```python
from build123d import *

# Parameters (mm, degrees)
F0_R     = 5.5
F0_R_2   = 3.25
F1_DEPTH = 30
F2_R     = 2.75
F2_R_2   = 1.75
F2_R_3   = 3.5
F2_R_4   = 8.25
F2_R_5   = 12.5
F3_DEPTH = 5
F5_DEPTH = 28
F7_DEPTH = 25
F8_SIZE  = 2


with BuildPart() as f1:
    # F0 (on Front) → F1 (new body)
    with BuildSketch(Plane.XZ):
        with Locations((28.2, -46.052)):
            Circle(F0_R)
        with Locations((28.2, -46.052)):
            Circle(F0_R_2, mode=Mode.SUBTRACT)
    extrude(amount=F1_DEPTH)



with BuildPart() as f1b:
    # F0 (on Front) → F1, piece 2 (new body)
    with BuildSketch(Plane.XZ):
        with Locations((-14.3, -46.052)):
            Circle(F0_R)
        with Locations((-14.3, -46.052)):
            Circle(F0_R_2, mode=Mode.SUBTRACT)
    extrude(amount=F1_DEPTH)


with BuildPart() as f1_1:
    add(f1.part)

    add(f1b.part)  # F3 merges F1b
    # F2 (on Front) → F3 (join)
    with BuildSketch(Plane.XZ):
        with BuildLine():
            Line((-47.5, 15), (-60, 15))
            ThreePointArc((-60, 15), (-75, 0), (-60, -15))
            Line((-60, -15), (-47.5, -15))
            ThreePointArc((-47.5, -15), (-43.9644660941, -16.4644660941), (-42.5, -20))
            Line((-42.5, -20), (-42.5, -60))
            Line((-42.5, -60), (42.5, -60))
            Line((42.5, -60), (42.5, 42.5))
            Line((42.5, 42.5), (-42.5, 42.5))
            Line((-42.5, 42.5), (-42.5, 20))
            ThreePointArc((-42.5, 20), (-43.9644660941, 16.4644660941), (-47.5, 15))
        make_face()
        with Locations((-37, -37)):
            Circle(F2_R, mode=Mode.SUBTRACT)
        with Locations((-53.9378221735, -10.5)):
            Circle(F2_R_2, mode=Mode.SUBTRACT)
        with Locations((-14.3, -46.052)):
            Circle(F2_R_3, mode=Mode.SUBTRACT)
        with Locations((28.2, -46.052)):
            Circle(F2_R_3, mode=Mode.SUBTRACT)
        with Locations((37, -37)):
            Circle(F2_R, mode=Mode.SUBTRACT)
        with Locations((-72.124355653, 0)):
            Circle(F2_R_2, mode=Mode.SUBTRACT)
        with Locations((-60, 0)):
            Circle(F2_R_4, mode=Mode.SUBTRACT)
        with Locations((-53.9378221735, 10.5)):
            Circle(F2_R_2, mode=Mode.SUBTRACT)
        with Locations((-37, 37)):
            Circle(F2_R, mode=Mode.SUBTRACT)
        Circle(F2_R_5, mode=Mode.SUBTRACT)
        with Locations((37, 37)):
            Circle(F2_R, mode=Mode.SUBTRACT)
    extrude(amount=F3_DEPTH)

    # F4 (on Front) → F5 (join)
    with BuildSketch(Plane.XZ):
        with BuildLine():
            Line((2, 19.8997487421), (2, 13.8564064606))
            ThreePointArc((2, 13.8564064606), (9.8994949366, 9.8994949366), (13.8564064606, 2))
            Line((13.8564064606, 2), (19.8997487421, 2))
            ThreePointArc((19.8997487421, 2), (14.1421356237, 14.1421356237), (2, 19.8997487421))
        make_face()
    extrude(amount=F5_DEPTH)

    # F6 (on Front) → F7 (join)
    with BuildSketch(Plane.XZ):
        with BuildLine():
            Line((28.2, -40.552), (-14.3, -40.552))
            ThreePointArc((-14.3, -40.552), (-8.8, -46.052), (-14.3, -51.552))
            Line((-14.3, -51.552), (28.2, -51.552))
            ThreePointArc((28.2, -51.552), (22.7, -46.052), (28.2, -40.552))
        make_face()
    extrude(amount=F7_DEPTH)

    # F8
    f8_edges = [f1_1.edges().sort_by_distance(p)[0] for p in [
        (-42.5, -2.5, 42.5),
        (42.5, -2.5, 42.5),
        (42.5, -2.5, -60),
        (-42.5, -2.5, -60),
    ]]
    chamfer(f8_edges, length=F8_SIZE)


solid = f1_1.part
```
Could you check a few things on this model? Use its own coordinates, in mm. A direction names the side the tool comes from. Round coordinates to 2 decimals unless told otherwise and drop trailing zeros. Loops run counter-clockwise (first coordinate to the right, second up) from the corner with the lowest first, then second, coordinate; pieces in that order, holes last. Notation, with made-up numbers: M 86,72 L 133,72 A20 ccw 133,98 Z; hole C 17.5,47.25 d7. An arc over 180 degrees is marked long. Answer as CSV lines item,"result".
1) Imagine slicing it at C-C on y = -9.5. List the corners of the cut face in (x, z) for me, and give its area (3 significant figures).
From the geometry:
outline,"M -14.3,-51.55 L 28.2,-51.55 A5.5 ccw 28.2,-40.55 L -14.3,-40.55 A5.5 ccw Z; M 2,13.86 A14 cw 13.86,2 L 19.9,2 A20 ccw 2,19.9 Z; hole C -14.3,-46.05 d6.5; hole C 28.2,-46.05 d6.5"
area,"632 mm^2"
2) Imagine slicing it at A-A on z = 37. List the corners of the cut face in (x, y) for me.
From the geometry:
outline,"M -42.5,-5 L -39.75,-5 L -39.75,0 L -42.5,0 Z; M -34.25,-5 L 34.25,-5 L 34.25,0 L -34.25,0 Z; M 39.75,-5 L 42.5,-5 L 42.5,0 L 39.75,0 Z"
3) Imagine slicing it at B-B on x = 0. List the corners of the cut face in (y, z) for me.
From the geometry:
outline,"M -25,-51.55 L -5,-51.55 L -5,-60 L 0,-60 L 0,-12.5 L -5,-12.5 L -5,-40.55 L -25,-40.55 Z; M -5,12.5 L 0,12.5 L 0,42.5 L -5,42.5 Z"
4) If I drill on probe 1 along Z at (x, y) = (37, -1.5); probe 2 along X at (y, z) = (-15.75, -43.5); probe 3 along Y at (x, z) = (-38, -11.5), over which ranges is the centre line in solid material (lowest first)?
From the geometry:
probe 1,"-60 to -39.75, -34.25 to 34.25, 39.75 to 42.5"
probe 2,"-19.17 to -16.31, -12.29 to 26.19, 30.21 to 33.07"
probe 3,"-5 to 0"
5) For pin 1 Ø3 at (x, z) = (-53.94, 10.5) entering from +Y; pin 2 Ø5.5 at (x, z) = (-53.94, -10.5) entering from -Y; pin 3 Ø4 at (y, z) = (-1.5, 30) entering from -X; pin 4 Ø5 at (y, z) = (-13, 4.5) entering from -X, each with a flat end and sliding along its axis, tell me the tip position at first contact or that it passes through.
From the geometry:
pin 1,"through"
pin 2,"y = -5"
pin 3,"x = -42.5"
pin 4,"x = 12.12"
6) Which directions (+Z, -Z, +X, -X, +Y, -Y) give clear straight access to the entire face, cutting with the end or side of a thin tool? Please do faces 4 (the flat face through (17, -16, 2)), 5 (the cylindrical face through (14.277, -16.339, 14.006)), 6 (the cylindrical face through (33.446, -20.103, -44.4)).
From the geometry:
face 4,"+X, -X, -Y"
face 5,"+Z, +X, -Y"
face 6,"-Y"
7) We'd pull the mould along X, two halves only. Please class faces 1 (the flat face through (7, -15, -51.552)), 2 (the cylindrical face through (-43.93, -2.46, 16.5)), 3 (the cylindrical face through (-39.027, -2.465, -35.141)): released by +X, released by -X, zero draft, split by the parting line, or undercut.
From the geometry:
face 1,"zero draft"
face 2,"released by -X"
face 3,"undercut"
8) Imagine slicing it at D-D on x = -38. List the corners of the cut face in (y, z) for me, and give its area (3 significant figures).
From the geometry:
outline,"M -5,-60 L 0,-60 L 0,-39.56 L -5,-39.56 Z; M -5,-34.44 L 0,-34.44 L 0,34.44 L -5,34.44 Z; M -5,39.56 L 0,39.56 L 0,42.5 L -5,42.5 Z"
area,"461 mm^2"
